Part model, mm, in its own coordinate system. A direction names the side the tool comes from. Coordinates: 2 decimals unless noted, no trailing zeros. Order: outer loops, then holes, each group sorted by start corner. A loop starts at its lowest first (then second) coordinate and runs counter-clockwise, first axis right, second up. Notation, with made-up numbers: M 21,10.5 L 71,10.5 A13 ccw 71,22.5 Z; hole C -36.75,25.5 d6. An arc over 180 degrees is marked long. Write item = value, one per line. Start each with the question number.
Autodesk Inventor part; units mm, degrees
ref_plane "YZ Plane" through (0, 0, 0) normal (1, 0, 0) x (0, 1, 0)
ref_plane "XZ Plane" through (0, 0, 0) normal (0, 1, 0) x (-1, 0, 0)
ref_plane "XY Plane" through (0, 0, 0) normal (0, 0, 1) x (1, 0, 0)
sketch "Sketch1" plane through (0, 0, 0) normal (1, 0, 0) x (0, 1, 0)
  circle A0 centre (0, 0) radius 38.1
  dimension "d0" = 76.2
extrude "Extrusion1" add sketch "Sketch1" along normal blind 76.2
sketch "Sketch2" plane through (76.2, 0, 0) normal (1, 0, 0) x (0, 0, -1)
  circle A0 centre (0, 0) radius 25.4
  dimension "d3" = 50.8
extrude "Extrusion2" cut sketch "Sketch2" against normal blind 152.4
sketch "Sketch3" plane through (76.2, 0, 0) normal (1, 0, 0) x (0, 0, -1)
  circle A0 centre (0, 0) radius 25.4
  circle A1 centre (0, 0) radius 25.4
  circle A2 centre (0.0066, 25.4) radius 3.81
  circle A3 centre (-17.9558, 17.9652) radius 3.81
  circle A4 centre (-25.4, 0.0066) radius 3.81
  circle A5 centre (-17.9652, -17.9558) radius 3.81
  circle A6 centre (-0.0066, -25.4) radius 3.81
  circle A7 centre (17.9558, -17.9652) radius 3.81
  circle A8 centre (25.4, -0.0066) radius 3.81
  circle A9 centre (17.9652, 17.9558) radius 3.81
  dimension "d6" = 7.62
  dimension "d9" = 360
extrude "Extrusion3" cut sketch "Sketch3" against normal blind 152.4 contours A0 A8 | A0 A8 | A9 A0 | A0 A9 | A7 A0 | A0 A7 | A2 A0 | A0 A2 | A6 A0 | A0 A6 | A3 A0 | A0 A3 | A5 A0 | A0 A5 | A4 A0 | A0 A4
Item 1: Cut at C-C, the plane x = 6. Write the cut outline in (y, z).
Item 2: Cut at A-A, the plane y = 0. Write the cut outline in (x, z).
Item 3: Wall check: line 1 along Y through (x, z) = (40.5, 3); line 2 along Y through (x, z) = (70, 13.5); line 3 along Z through (x, y) = (41, 10.5). Give the ranges that are in metal, low to high. Write a range as [from, to].
Item 4: Flat gauge pins, fed straight in: pin 1 (12 mm diameter, centred on x = 41.5, z = -14, fed in from +Y); pin 2 (2 mm diameter, centred on x = 12.5, z = -12.5, fed in from -Y); pin 3 (12 mm diameter, centred on x = 57, z = 10.5, fed in from -Y). Where does each tip first touch, or does it go through?
Item 5: Pull direction Z, two halves, no side cores. Call faces 3 (the flat face through (0, 8, -25)), 4 (the cylindrical face through (38.633, 23.502, 9.634)), 5 (the cylindrical face through (38.63, -20.72, -20.59)): pulls with the +Z half, pulls with the -Z half, needs draft (parallel to the pull), parting line crosses it, or undercut.
Item 6: 3-axis set-ups, long thin cutter, end or side, ignore diameter. For faces 1 (the cylindrical face through (38.63, -9.81, -23.43)), 2 (the flat face through (76.2, 8, -25)): which of +Z, -Z, +X, -X, +Y, -Y reach the whole face in a straight line?
Filled sheet:
q1.outline = C 0,0 d76.2; hole M -25.12,-3.79 A25.4 ccw -20.45,-15.07 A3.81 ccw long -15.08,-20.44 A25.4 ccw -3.81,-25.11 A3.81 ccw long 3.79,-25.12 A25.4 ccw 15.07,-20.45 A3.81 ccw long 20.44,-15.08 A25.4 ccw 25.11,-3.81 A3.81 ccw long 25.12,3.79 A25.4 ccw 20.45,15.07 A3.81 ccw long 15.08,20.44 A25.4 ccw 3.81,25.11 A3.81 ccw long -3.79,25.12 A25.4 ccw -15.07,20.45 A3.81 ccw long -20.44,15.08 A25.4 ccw -25.11,3.81 A3.81 ccw long Z
q2.outline = M 0,-38.1 L 76.2,-38.1 L 76.2,-29.21 L 0,-29.21 Z; M 0,29.21 L 76.2,29.21 L 76.2,38.1 L 0,38.1 Z
q3.line_1 = [-37.98, -27.76], [27.74, 37.98]
q3.line_2 = [-35.63, -21.52], [21.52, 35.63]
q3.line_3 = [-36.62, -23.13], [23.13, 36.62]
q4.pin_1 = 37.25
q4.pin_2 = -36.32
q4.pin_3 = -37.83
q5.face_3 = needs draft
q5.face_4 = undercut
q5.face_5 = undercut
q6.face_1 = +X, -X
q6.face_2 = +Z, -Z, +X, +Y, -Y
